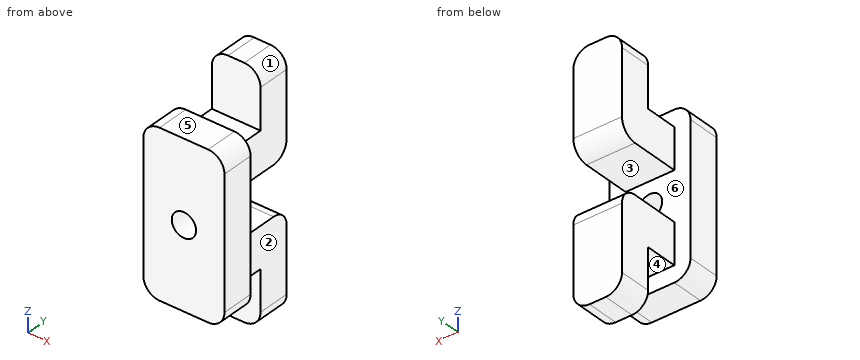
Autodesk Inventor part; units mm, degrees
ref_plane "YZ Plane" through (0, 0, 0) normal (1, 0, 0) x (0, 1, 0)
ref_plane "XZ Plane" through (0, 0, 0) normal (0, 1, 0) x (-1, 0, 0)
ref_plane "XY Plane" through (0, 0, 0) normal (0, 0, 1) x (1, 0, 0)
sketch "Sketch1" plane through (0, 0, 0) normal (0, 1, 0) x (-1, 0, 0)
  line L0 (0, 0) -> (10, 0)
  line L1 (10, 0) -> (10, 20)
  line L2 (10, 20) -> (0, 20)
  line L3 (0, 20) -> (0, 0)
  dimension "d0" = 10
  dimension "d1" = 20
extrude "Extrusion1" add sketch "Sketch1" along normal blind 4
sketch "Sketch2" plane through (0, 4, 0) normal (0, 1, 0) x (1, 0, 0)
  line L0 (-8, -18) -> (-2, -18)
  line L1 (-2, -18) -> (-2, -13)
  line L2 (-2, -13) -> (-8, -13)
  line L3 (-8, -13) -> (-8, -18)
  line L4 (-8, -2) -> (-2, -2)
  line L5 (-2, -2) -> (-2, -7)
  line L6 (-2, -7) -> (-8, -7)
  line L7 (-8, -7) -> (-8, -2)
  point P0 (0, 0)
  dimension "d4" = 6
  dimension "d5" = 5
  dimension "d6" = 5
extrude "Extrusion2" add sketch "Sketch2" along normal blind 8
sketch "Sketch3" plane through (-8, 4, 18) normal (0, 0, 1) x (1, 0, 0)
  line L0 (0, 0) -> (0, 8)
  line L1 (6, 8) -> (0, 8)
  line L2 (0, 8) -> (0, 4)
  line L3 (0, 4) -> (6, 4)
  line L4 (6, 4) -> (6, 8)
  point P0 (8, -4)
  point P1 (0, 8)
  dimension "d9" = 4
extrude "Extrusion3" add sketch "Sketch3" along normal blind 7
sketch "Sketch4" plane through (-2, 4, 2) normal (0, 0, -1) x (-1, 0, 0)
  line L0 (0, 8) -> (6, 8)
  line L1 (0, 8) -> (6, 8)
  line L2 (6, 8) -> (6, 4)
  line L3 (6, 4) -> (0, 4)
  line L4 (0, 4) -> (0, 8)
  point P0 (-2, -4)
  dimension "d12" = 4
extrude "Extrusion4" add sketch "Sketch4" along normal blind 7
fillet "Fillet1" radius 2 8 edges at (-2, 10, -5) (-8, 10, -5) (-2, 10, 25) (-8, 10, 25) (0, 2, 20) (0, 2, 0) (-10, 2, 0) (-10, 2, 20)
sketch "Sketch5" plane through (0, 4, 0) normal (0, 1, 0) x (1, 0, 0)
  circle A0 centre (-5, -10) radius 1.5
  point P0 (0, 0)
  dimension "d16" = 3
extrude "Extrusion5" cut sketch "Sketch5" against normal blind 7
fillet "Fillet2" radius 2 2 edges at (-5, 12, 13) (-5, 12, 7)
properties part number "PlatformSlider"
Could you check a few things on this model? Use its own coordinates, in mm. Face numbers are marked on the shaded views. A direction names the side the tool comes from. Coordinates: 2 decimals unless noted, no trailing zeros. Write each loop counter-clockwise with the first axis right and the second up, starting at its lowest first coordinate (ties: lowest second). Pieces come first, ordered by that corner, then holes. Notation, with made-up numbers: (26.25, 13) - (75.25, 13) arc R27 ccw to (75.25, 47) - close; hole circle Ø8 at (79.5, 85). An arc over 180 degrees is marked (long way). Put each result on its own line as item: value. Start each with the question number.
Q1. Please list where these lines run through material, in increasing order: L1, parallel to Z at x = -7.75, y = 6.5; L2, parallel to X at y = 3.05, z = 10; L3, parallel to Y at x = -6.75, z = 19.75.
Q2. I want a section at A-A on y = 8.75. Write out the boundary of the cut face in (x, z).
Q3. I want a section at C-C on z = 3. Write out the boundary of the cut face in (x, y), plus the area to 3 significant figures.
Q4. Thinking about a two-plate mould opening in Z: for the marked faces 1, 2 and 3, which applies, pulls with the +Z half, pulls with the -Z half, needs draft (parallel to the pull), parting line crosses it, or undercut?
Q5. I want a section at B-B on x = -5. Write out the boundary of the cut face in (y, z).
Q6. Which directions (+Z, -Z, +X, -X, +Y, -Y) give clear straight access to the entire face, cutting with the end or side of a thin tool? Please do the marked faces 4, 5 and 6.
Q7. I'm going to push flat-ended pins straight in: P1, Ø1.5, axis at x = -8, y = 2, coming from the -Z side; P2, Ø6.5, axis at y = 7.5, z = 1.5, coming from the -X side; P3, Ø1.8, axis at x = -5, z = 10, coming from the -Y side; P4, Ø6, axis at x = -8.5, y = 3, coming from the +Z side. Where does each tip first touch, or does it pass through?
Q8. I want a section at D-D on z = 10. Write out the boundary of the cut face in (x, y), plus the area to 3 significant figures.
Checks:
1. L1: 2 to 7, 13 to 18
1. L2: -10 to -6.5, -3.5 to 0
1. L3: 0 to 4, 8 to 12
2. outline: (-8, -3) arc R2 ccw to (-6, -5) - (-4, -5) arc R2 ccw to (-2, -3) - (-2, 7) - (-8, 7) - close; (-8, 13) - (-2, 13) - (-2, 23) arc R2 ccw to (-4, 25) - (-6, 25) arc R2 ccw to (-8, 23) - close
3. outline: (-10, 0) - (0, 0) - (0, 4) - (-2, 4) - (-2, 12) - (-8, 12) - (-8, 4) - (-10, 4) - close
3. area: 88.0 mm²
4. face 1: pulls with the +Z half
4. face 2: needs draft
4. face 3: undercut
5. outline: (0, 0) - (4, 0) - (4, 2) - (8, 2) - (8, -5) - (12, -5) - (12, 5) arc R2 ccw to (10, 7) - (4, 7) - (4, 8.5) - (0, 8.5) - close; (0, 11.5) - (4, 11.5) - (4, 13) - (10, 13) arc R2 ccw to (12, 15) - (12, 25) - (8, 25) - (8, 18) - (4, 18) - (4, 20) - (0, 20) - close
6. face 4: -Z, +X, -X
6. face 5: +Z, +X, -X, -Y
6. face 6: none
7. P1: z = 0
7. P2: x = -8
7. P3: through
7. P4: z = 20
8. outline: (-10, 0) - (-6.5, 0) - (-6.5, 4) - (-10, 4) - close; (-3.5, 0) - (0, 0) - (0, 4) - (-3.5, 4) - close
8. area: 28.0 mm²
